Autodesk Inventor part; units mm, degrees
ref_plane "YZ Plane" through (0, 0, 0) normal (1, 0, 0) x (0, 1, 0)
ref_plane "XZ Plane" through (0, 0, 0) normal (0, 1, 0) x (-1, 0, 0)
ref_plane "XY Plane" through (0, 0, 0) normal (0, 0, 1) x (1, 0, 0)
sketch "Sketch1" plane through (0, 0, 0) normal (0, 0, 1) x (1, 0, 0)
  circle A0 centre (0, 0) radius 43
  circle A1 centre (0, 0) radius 8
  circle A2 centre (0, 25) radius 8
  circle A3 centre (-17.6777, 17.6777) radius 8
  circle A4 centre (-25, 0) radius 8
  circle A5 centre (-17.6777, -17.6777) radius 8
  circle A6 centre (0, -25) radius 8
  circle A7 centre (17.6777, -17.6777) radius 8
  circle A8 centre (25, 0) radius 8
  circle A9 centre (17.6777, 17.6777) radius 8
  dimension "diameter" = 16
  dimension "d2" = 16
  dimension "d5" = 360
  dimension "d7" = 25
  dimension "d28" = 86
extrude "Extrusion1" add sketch "Sketch1" along normal blind 12
extrude "Extrusion2" add sketch "Sketch1" along normal blind 2 contours A2
extrude "Extrusion3" add sketch "Sketch1" along normal blind 3 contours A9
extrude "Extrusion4" add sketch "Sketch1" along normal blind 4 contours A8
extrude "Extrusion5" add sketch "Sketch1" along normal blind 5 contours A7
extrude "Extrusion6" add sketch "Sketch1" along normal blind 6 contours A6
extrude "Extrusion7" add sketch "Sketch1" along normal blind 7 contours A5
extrude "Extrusion8" add sketch "Sketch1" along normal blind 8 contours A4
extrude "Extrusion9" add sketch "Sketch1" along normal blind 9 contours A3
extrude "Extrusion10" add sketch "Sketch1" along normal blind 10 contours A1
sketch "Sketch2" plane through (0, 0, 12) normal (0, 0, 1) x (1, 0, 0)
  line L0 (-5.8774, 39.105) -> (5.7366, 39.105) construction
  line L1 (5.7366, 39.105) -> (5.7366, 35.936) construction
  line L2 (5.7366, 35.936) -> (-5.8774, 35.936) construction
  line L3 (-5.8774, 35.936) -> (-5.8774, 39.105) construction
  point P0 (0, 0)
emboss "Emboss1" [suppressed]
chamfer "Chamfer1" distance 1 angle 45 1 edges at (-43, 0, 12)
equation "\"d2\" = diameter"
properties part number "Diameter_16mm"
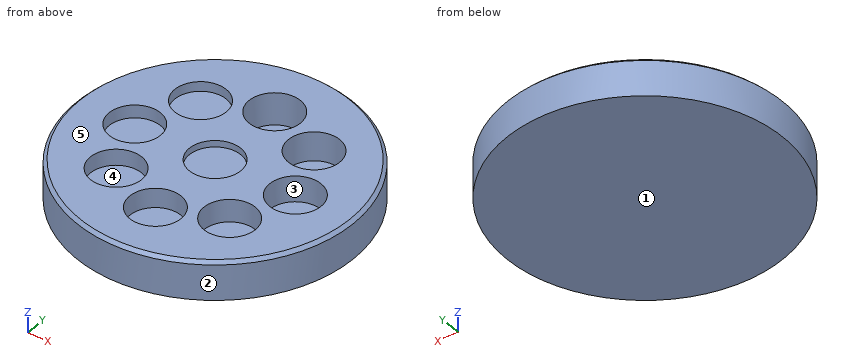
Geometry: final body of the model. Coordinates: model frame, mm. Face numbers are marked on the shaded views. A direction names the side the tool comes from. Give positions to 0.01 mm unless a question says otherwise; leave off trailing zeros. Loops run counter-clockwise (first coordinate to the right, second up) from the corner with the lowest first, then second, coordinate; pieces in that order, holes last. Notation, with made-up numbers: (-24.5, 83) - (5.5, 83) arc R12 cw to (5.5, 94) - close; hole circle Ø1 at (-22, 49). An arc over 180 degrees is marked (long way). Answer as CSV lines item,"result". Start each with the question number.
1. Reachability of the marked faces 4 and 5 from +Z, -Z, +X, -X, +Y, -Y: full face, straight path, thin tool, end or side. Return the list, or none.
2. Section B-B, the plane y = 0. Return loops of the section in (x, z), plus the area to 3 significant figures.
3. Pin query (flat end, axial travel): P1, Ø9.5, axis at x = 17.68, y = 17.68, coming from the +Z side; P2, Ø9.5, axis at x = -17.68, y = -17.68, coming from the +Z side; P3, Ø3, axis at y = -19.5, z = 10.5, coming from the -X side. Return the tip coordinate at first contact, or that it passes through.
4. Ray query, L1, parallel to Y at x = 0, z = 8.75; L2, parallel to Y at x = 0, z = 10.75; L3, parallel to X at y = 22, z = 8. Return the intervals inside material, ascending.
5. Section A-A, the plane x = 0. Return loops of the section in (y, z), plus the area to 3 significant figures.
6. Draft query along X for the marked faces 1, 2 and 3. Return one class per face: released by +X, released by -X, zero draft, split by the parting line, or undercut.
Answers:
1,face 4,"+Z"
1,face 5,"+Z, +X, -X, +Y, -Y"
2,outline,"(-43, 0) - (43, 0) - (43, 11) - (42, 12) - (33, 12) - (33, 4) - (17, 4) - (17, 12) - (8, 12) - (8, 10) - (-8, 10) - (-8, 12) - (-17, 12) - (-17, 8) - (-33, 8) - (-33, 12) - (-42, 12) - (-43, 11) - close"
2,area,"807 mm2"
3,P1,"stops at z = 3"
3,P2,"stops at z = 7"
3,P3,"stops at x = -39.05"
4,L1,"y = -43 to -33, -17 to 17, 33 to 43"
4,L2,"y = -43 to -33, -17 to -8, 8 to 17, 33 to 43"
4,L3,"x = -36.95 to -7.42, 7.42 to 10.95, 24.41 to 36.95"
5,outline,"(-43, 0) - (43, 0) - (43, 11) - (42, 12) - (33, 12) - (33, 2) - (17, 2) - (17, 12) - (8, 12) - (8, 10) - (-8, 10) - (-8, 12) - (-17, 12) - (-17, 6) - (-33, 6) - (-33, 12) - (-42, 12) - (-43, 11) - close"
5,area,"743 mm2"
6,face 1,"zero draft"
6,face 2,"split by the parting line"
6,face 3,"undercut"
